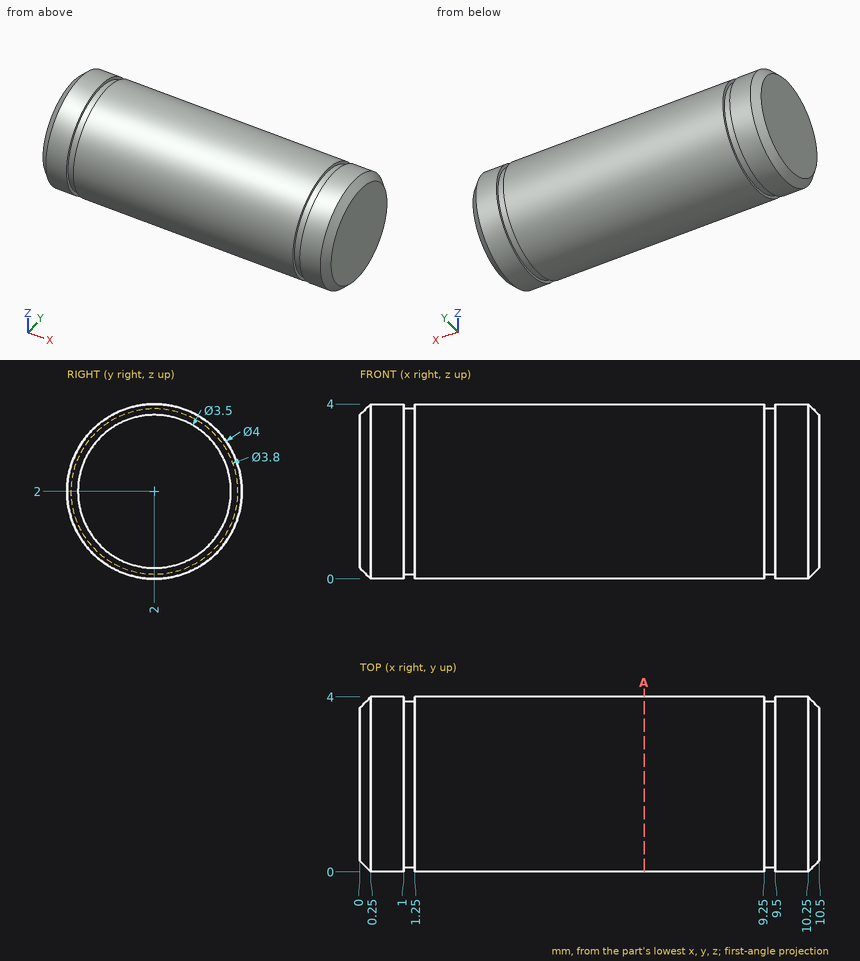
Verification items for this drawing (mm, ordinates from the low corner). Round coordinates to 2 decimals unless told otherwise and drop trailing zeros. Order: outer loops, then holes, each group sorted by start corner. A loop starts at its lowest first (then second) coordinate and runs counter-clockwise, first axis right, second up.
1) Depth check by flat-ended pin: pin 1 (1.5 mm diameter, centred on x = 5.5, z = 1, fed in from -Y). Enter the tip coordinate at first touch or a pass-through.
Geometry says:
pin 1: stops at y = 0.02
2) Material ranges on line 1 (Y direction, x = 5, z = 1.9); line 2 (Y direction, x = 8.25, z = 0.4); line 3 (Z direction, x = 7.25, y = 2.95), recorded low to high.
Geometry says:
line 1: y = 0 to 4
line 2: y = 0.8 to 3.2
line 3: z = 0.24 to 3.76
3) Cross-section at A-A, the plane x = 6.5. Record the cut outline in (y, z), plus the area to 3 significant figures.
Geometry says:
outline: circle Ø4 at (2, 2)
area: 12.6 mm2
